from build123d import *

# Parameters (mm, degrees)
F0_W     = 200
F0_H     = 36
F1_DEPTH = 18
F2_R     = 15
F3_DEPTH = 3
F4_W     = 10
F4_H     = 16
F4_R     = 2.25
F5_DEPTH = 8


with BuildPart() as f1:
    # F0 (on Top) → F1 (new body)
    with BuildSketch(Plane.XY):
        Rectangle(F0_W, F0_H)
    extrude(amount=F1_DEPTH)

    # F2 (on face) → F3 (cut)
    with BuildSketch(Plane.XY.offset(18)):
        with Locations((-20, 0)):
            Circle(F2_R)
        with Locations((40, 0)):
            Circle(F2_R)
    extrude(amount=-F3_DEPTH, mode=Mode.SUBTRACT)

    # F4 (on face) → F5 (join)
    with BuildSketch(Plane.XY.offset(18)):
        with Locations((-105, 0)):
            Rectangle(F4_W, F4_H)
        with Locations((-104.25, 0)):
            Circle(F4_R, mode=Mode.SUBTRACT)
        with Locations((105, 0)):
            Rectangle(F4_W, F4_H)
        with Locations((104.25, 0)):
            Circle(F4_R, mode=Mode.SUBTRACT)
    extrude(amount=-F5_DEPTH)


solid = f1.part
Work out the finished part from the listing and answer in its coordinate system (mm). A direction names the side the tool comes from. Give positions to 0.01 mm unless a question says otherwise; leave off trailing zeros. Order: outer loops, then holes, each group sorted by start corner. A loop starts at its lowest first (then second) coordinate and runs counter-clockwise, first axis right, second up. Notation, with made-up numbers: (83, 5.5) -> (105, 5.5) arc R25 cw to (105, 21.5) -> close; hole circle Ø9 at (37.25, 18.5). An arc over 180 degrees is marked (long way). One line per item, written item: value.
Item 1: Straight lines are drawn through the part: probe 1 along Y at (x, z) = (40, 17.2); probe 2 along X at (y, z) = (-13.5, 14.25); probe 3 along Z at (x, y) = (49.5, -11). For each, find the intervals that lie inside material, in ascending order.
Answer sheet:
probe 1: -18 to -15, 15 to 18
probe 2: -100 to 100
probe 3: 0 to 15
Item 2: Find section B-B, the plane x = 104.25. Give the vertices of the cut face in (y, z).
Answer sheet:
outline: (-8, 10) -> (-2.25, 10) -> (-2.25, 18) -> (-8, 18) -> close; (2.25, 10) -> (8, 10) -> (8, 18) -> (2.25, 18) -> close
Item 3: Determine the mould class of faces 1 (the flat face through (-2, 0, 18)), 2 (the flat face through (-1, -18, 9)), 3 (the cylindrical face through (-102.17, -0.86, 14.06)), 4 (the flat face through (40, 0, 15)) for opening direction Y: released by +Y, released by -Y, zero draft, split by the parting line, or undercut.
Answer sheet:
face 1: zero draft
face 2: released by -Y
face 3: undercut
face 4: undercut
Item 4: Find section C-C, the plane x = 40. Give the vertices of the cut face in (y, z).
Answer sheet:
outline: (-18, 0) -> (18, 0) -> (18, 18) -> (15, 18) -> (15, 15) -> (-15, 15) -> (-15, 18) -> (-18, 18) -> close
Item 5: Find section D-D, the plane z = 12. Give the vertices of the cut face in (x, y), plus the area to 3 significant figures.
Answer sheet:
outline: (-110, -8) -> (-100, -8) -> (-100, -18) -> (100, -18) -> (100, -8) -> (110, -8) -> (110, 8) -> (100, 8) -> (100, 18) -> (-100, 18) -> (-100, 8) -> (-110, 8) -> close; hole circle Ø4.5 at (-104.25, 0); hole circle Ø4.5 at (104.25, 0)
area: 7,490 mm²
Item 6: Flat-ended cylindrical pins translate along their axes: P1, Ø9, axis at x = 106.5, z = 13, coming from the -Y side; P2, Ø9, axis at x = -105, z = 15.5, coming from the +Y side; P3, Ø9, axis at x = -17.5, y = -6.5, coming from the +Z side. Find the tip coordinate at first contact, or state that the pin passes through.
Answer sheet:
P1: y = -8
P2: y = 8
P3: z = 15
Item 7: Find section A-A, the plane y = 0. Give the vertices of the cut face in (x, z).
Answer sheet:
outline: (-110, 10) -> (-106.5, 10) -> (-106.5, 18) -> (-110, 18) -> close; (-102, 10) -> (-100, 10) -> (-100, 0) -> (100, 0) -> (100, 10) -> (102, 10) -> (102, 18) -> (55, 18) -> (55, 15) -> (25, 15) -> (25, 18) -> (-5, 18) -> (-5, 15) -> (-35, 15) -> (-35, 18) -> (-102, 18) -> close; (106.5, 10) -> (110, 10) -> (110, 18) -> (106.5, 18) -> close
Item 8: A tool of negligible diameter and unlimited length cuts with its end or side. For faces 5 (the cylindrical face through (25.015, 0.66, 16.521)), 6 (the flat face through (105, -8, 14)), 7 (the flat face through (-105, -8, 14)), from which of +Z, -Z, +X, -X, +Y, -Y can it reach the whole face along a straight path? Write none if from no direction.
Answer sheet:
face 5: +Z
face 6: +Z, -Z, +X, -Y
face 7: +Z, -Z, -X, -Y
